Model file for the job. Use its own axes, mm. A direction names the side the tool comes from. Round coordinates to 2 decimals unless told otherwise and drop trailing zeros. Write each loop counter-clockwise with the first axis right and the second up, starting at its lowest first coordinate (ties: lowest second). Pieces come first, ordered by that corner, then holes. Notation, with made-up numbers: (27.25, -27.75) - (35.25, -27.75) arc R25 cw to (35.25, -8.75) - close; hole circle Ø4 at (12, 2.25). An arc over 180 degrees is marked (long way). Answer as a JSON object with one key per item and string values. Group by question number.
from build123d import *

# Parameters (mm, degrees)
BOSS_EXTRUDE1_DEPTH = 60
SKETCH2_W           = 18
SKETCH2_H           = 3
BOSS_EXTRUDE2_DEPTH = 10
CHAMFER1_SIZE       = 10.069195574
CHAMFER1_SIZE_2     = 12
FILLET1_R           = 5


with BuildPart() as part:
    # Sketch1 → Boss-Extrude1 (new body)
    with BuildSketch(Plane.XY):
        Polygon((0, 0), (0, 30), (20.5, 30), (20.5, 0), (69.5, 0), (69.5, 6), (29.5, 6), (29.5, 36), (-9, 36), (-9, 0), align=None)
    extrude(amount=BOSS_EXTRUDE1_DEPTH)

    # Sketch2 → Boss-Extrude2 (add)
    with BuildSketch(Plane(origin=(0, 6, 0), x_dir=(1, 0, 0), z_dir=(0, 1, 0))):
        with Locations((38.5, -1.5)):
            Rectangle(SKETCH2_W, SKETCH2_H)
        Polygon((50.5, 0), (47.5, 0), (47.5, -3), (47.5, -28.5), (47.5, -31.5), (47.5, -57), (47.5, -60), (69.5, -60), (69.5, -57), (50.5, -57), align=None)
        with Locations((38.5, -30)):
            Rectangle(SKETCH2_W, SKETCH2_H)
        with Locations((38.5, -58.5)):
            Rectangle(SKETCH2_W, SKETCH2_H)
    extrude(amount=BOSS_EXTRUDE2_DEPTH)

    # Chamfer1
    # the kernel refuses this chamfer: 12, 10.069195574 mm, written as the material it adds along each edge
    with BuildSketch(Plane(origin=(29.5, 6, 31.5), x_dir=(0, 0.9993728857116145, -0.03540953691366269), z_dir=(1, 0, 0))) as chamfer1_piece_1_section:
        Polygon((CHAMFER1_SIZE * 0.999372885724, CHAMFER1_SIZE * 0.0354095369141), (-CHAMFER1_SIZE_2 * 0.0354095369137, CHAMFER1_SIZE_2 * 0.999372885712), (0, 0), align=None)
    chamfer1_piece_1 = extrude(amount=18, mode=Mode.PRIVATE)
    chamfer1_piece_1 = split(chamfer1_piece_1, bisect_by=Plane(origin=(38.5, 16, 35.487012509), z_dir=(0, -1, 0)), keep=Keep.TOP, mode=Mode.PRIVATE)
    add(chamfer1_piece_1)
    with BuildSketch(Plane(origin=(29.5, 6, 3), x_dir=(0, -0.024939322090234344, 0.9996889667359941), z_dir=(1, 0, 0))) as chamfer1_piece_2_section:
        Polygon((CHAMFER1_SIZE_2 * 0.999688966736, -CHAMFER1_SIZE_2 * 0.0249393220902), (-CHAMFER1_SIZE * 0.0249393220905, -CHAMFER1_SIZE * 0.999688966749), (0, 0), align=None)
    chamfer1_piece_2 = extrude(amount=18, mode=Mode.PRIVATE)
    chamfer1_piece_2 = split(chamfer1_piece_2, bisect_by=Plane(origin=(38.5, 16, 6.987012509), z_dir=(0, -1, 0)), keep=Keep.TOP, mode=Mode.PRIVATE)
    add(chamfer1_piece_2)

    # Fillet1
    fillet1_edges = [part.edges().sort_by_distance(p)[0] for p in [
        (-9, 36, 30),
        (29.5, 36, 30),
    ]]
    fillet(fillet1_edges, radius=FILLET1_R)


solid = part.part
(1) Slice it at D-D (y = 15). Write the cut outline in (x, z).
(2) Slice it at B-B (x = 40). Write the cut outline in (y, z), then the cut area to 3 significant figures.
(3) Pull direction X, two halves, no side cores. Call faces 1 (the flat face through (38.374, 10.93, 9.125)), 2 (the flat face through (-9, 16, 30)), 3 (the flat face through (-5, 0, 30)), 4 (the flat face through (47.5, 11, 18)): pulls with the +X half, pulls with the -X half, needs draft (parallel to the pull), parting line crosses it, or undercut.
(4) Drill centre lines: line 1 (X direction, y = 14, z = 51.5); line 2 (X direction, y = 20, z = 39); line 3 (X direction, y = 5, z = 11). Where is each one in solid material? Low to high. Write a range as from..to.
(5) Slice it at C-C (z = 55). Write the cut outline in (x, y), then the cut area to 3 significant figures.
(6) Slice it at A-A (y = 3.5). Write the cut outline in (x, z), then the cut area to 3 significant figures.
(7) Flat gauge pins, fed straight in: pin 1 (11 mm diameter, centred on x = 36, z = 53, fed in from +Y); pin 2 (6 mm diameter, centred on y = 16, z = 44, fed in from +X); pin 3 (3 mm diameter, centred on x = 60.5, y = 12.5, fed in from -Z). Where does each tip first touch, or does it go through?
(8) 3-axis set-ups, long thin cutter, end or side, ignore diameter. For faces 5 (the flat face through (38, 11, 28.5)), 6 (the flat face through (0, 15, 30)), 7 (the flat face through (50.5, 11, 29)): which of +Z, -Z, +X, -X, +Y, -Y reach the whole face in a straight line?
Answer:
{
 "1": {"outline": "(-9, 0) - (0, 0) - (0, 60) - (-9, 60) - close; (20.5, 0) - (50.5, 0) - (50.5, 57) - (69.5, 57) - (69.5, 60) - (20.5, 60) - close; hole (29.5, 4.27) - (47.5, 4.27) - (47.5, 28.5) - (29.5, 28.5) - close; hole (29.5, 32.77) - (47.5, 32.77) - (47.5, 57) - (29.5, 57) - close"},
 "2": {"outline": "(0, 0) - (16, 0) - (16, 3.08) - (6, 15) - (6, 28.5) - (16, 28.5) - (16, 31.58) - (6, 43.5) - (6, 57) - (16, 57) - (16, 60) - (0, 60) - close", "area": "571 mm²"},
 "3": {"face 1": "undercut", "face 2": "pulls with the -X half", "face 3": "needs draft", "face 4": "undercut"},
 "4": {"line 1": "-9..0, 20.5..29.5, 47.5..50.5", "line 2": "-9..0, 20.5..29.5", "line 3": "-9..0, 20.5..69.5"},
 "5": {"outline": "(-9, 0) - (0, 0) - (0, 30) - (20.5, 30) - (20.5, 0) - (69.5, 0) - (69.5, 6) - (50.5, 6) - (50.5, 16) - (47.5, 16) - (47.5, 6) - (29.5, 6) - (29.5, 31) arc R5 ccw to (24.5, 36) - (-4, 36) arc R5 ccw to (-9, 31) - close", "area": "1,030 mm²"},
 "6": {"outline": "(-9, 0) - (0, 0) - (0, 60) - (-9, 60) - close; (20.5, 0) - (69.5, 0) - (69.5, 60) - (20.5, 60) - close", "area": "3,480 mm²"},
 "7": {"pin 1": "y = 16", "pin 2": "x = 50.5", "pin 3": "z = 57"},
 "8": {"face 5": "+Y", "face 6": "+Z, -Z, -Y", "face 7": "-Z, +X, +Y"}
}
